Input: part model. Units: mm. Frame: model coordinates. A direction names the side the tool comes from. Give positions to 0.01 mm unless a question says otherwise; leave off trailing zeros. Write each loop counter-clockwise with the first axis right and the second up, starting at its lowest first coordinate (ties: lowest second). Pieces come first, ordered by that corner, then holes. Notation, with made-up numbers: (-5.75, 60) -> (25.25, 60) arc R22 cw to (25.25, 89) -> close; hole circle Ø5 at (14, 12.5). An arc over 180 degrees is marked (long way). Return JSON: item names as keys, results as strings. Group by question number.
Item 1: Mould query, pull axis Z, two halves, no side actions, for faces 5 (the face through (38, 35, 25.4)), 6 (the face through (41, 35, 33.02)), 7 (the face through (0, 34, 0)), 8 (the face through (12, -38.1, 7)). Classes: released by +Z, released by -Z, zero draft, split by the parting line, or undercut.
Item 2: Section A-A, the plane z = 22.5. Return loops of the section in (x, y).
Item 3: Line query: line 1 (X direction, y = -26.5, z = 4); line 2 (Y direction, x = -17, z = 3). Output: solid intervals per line, ascending. Write a range as [from, to].
Item 4: Section D-D, the plane y = 33. Return loops of the section in (x, z).
Item 5: Section C-C, the plane z = 3. Return loops of the section in (x, y).
Item 6: Section B-B, the plane x = 25. Return loops of the section in (y, z), then the cut area to 3 significant figures.
Item 7: Pin query (flat end, axial travel): P1, Ø1.9, axis at y = -35, z = 14, coming from the -X side; P2, Ø1, axis at y = 24.5, z = 10, coming from the -X side; P3, Ø5, axis at y = -36, z = 27.5, coming from the -X side; P4, Ø1.9, axis at x = 49, y = -11.5, coming from the +Z side. Return the tip coordinate at first contact, or that it passes through.
Item 8: Set-up query: faces 1 (the face through (-1, -31.75, 4)), 2 (the face through (46, 31.75, 23)), 3 (the face through (44.45, -35, 16)), 4 (the face through (31.75, -35, 29)). Return all of +Z, -Z, +X, -X, +Y, -Y with unobstructed straight access to the full face (end or side cutting, diameter ignored); none if empty.
from build123d import *

# Parameters (mm, degrees)
F0_W     = 88.9
F0_H     = 63.5
F1_DEPTH = 7.62
F2_W     = 6.35
F2_H     = 6.35
F3_DEPTH = 25.4
F4_W     = 6.35
F4_H     = 7.62
F5_DEPTH = 12.7
F6_W     = 6.35
F6_H     = 7.62
F7_DEPTH = 12.7


with BuildPart() as f1:
    # F0 (on Top) → F1 (new body)
    with BuildSketch(Plane.XY):
        Polygon((50.8, 38.1), (-50.8, 38.1), (-50.8, -38.1), (50.8, -38.1), (50.8, 4.614057), align=None)
        Rectangle(F0_W, F0_H, mode=Mode.SUBTRACT)
    extrude(amount=F1_DEPTH)

    # F2 (on face) → F3 (join)
    with BuildSketch(Plane.XY.offset(7.62)):
        with Locations((47.625, -34.925)):
            Rectangle(F2_W, F2_H)
        with Locations((47.625, 34.925)):
            Rectangle(F2_W, F2_H)
    extrude(amount=F3_DEPTH)

    # F4 (on face) → F5 (join)
    with BuildSketch(Plane(origin=(44.45, 0, 0), x_dir=(0, -1, 0), z_dir=(-1, 0, 0))):
        with Locations((-34.925, 29.21)):
            Rectangle(F4_W, F4_H)
    extrude(amount=F5_DEPTH)

    # F6 (on face) → F7 (join)
    with BuildSketch(Plane(origin=(44.45, 0, 0), x_dir=(0, -1, 0), z_dir=(-1, 0, 0))):
        with Locations((34.925, 29.21)):
            Rectangle(F6_W, F6_H)
    extrude(amount=F7_DEPTH)


solid = f1.part
Answer below:
{
 "1": {"face 5": "undercut", "face 6": "released by +Z", "face 7": "released by -Z", "face 8": "zero draft"},
 "2": {"outline": "(44.45, -38.1) -> (50.8, -38.1) -> (50.8, -31.75) -> (44.45, -31.75) -> close; (44.45, 31.75) -> (50.8, 31.75) -> (50.8, 38.1) -> (44.45, 38.1) -> close"},
 "3": {"line 1": "x = [-50.8, -44.45], [44.45, 50.8]", "line 2": "y = [-38.1, -31.75], [31.75, 38.1]"},
 "4": {"outline": "(-50.8, 0) -> (50.8, 0) -> (50.8, 33.02) -> (31.75, 33.02) -> (31.75, 25.4) -> (44.45, 25.4) -> (44.45, 7.62) -> (-50.8, 7.62) -> close"},
 "5": {"outline": "(-50.8, -38.1) -> (50.8, -38.1) -> (50.8, 38.1) -> (-50.8, 38.1) -> close; hole (-44.45, -31.75) -> (44.45, -31.75) -> (44.45, 31.75) -> (-44.45, 31.75) -> close"},
 "6": {"outline": "(-38.1, 0) -> (-31.75, 0) -> (-31.75, 7.62) -> (-38.1, 7.62) -> close; (31.75, 0) -> (38.1, 0) -> (38.1, 7.62) -> (31.75, 7.62) -> close", "area": "96.8 mm2"},
 "7": {"P1": "stops at x = 44.45", "P2": "passes through", "P3": "stops at x = 31.75", "P4": "stops at z = 7.62"},
 "8": {"face 1": "+Z, -Z", "face 2": "+Z, +X, -X", "face 3": "-X, +Y, -Y", "face 4": "+Z, -X, +Y, -Y"}
}
